Check sheet for the drawn part. Datum: minimum x, y, z corner. Units: mm. A direction names the side the tool comes from. Coordinates: 2 decimals unless noted, no trailing zeros. Order: outer loops, then holes, each group sorted by start corner. A loop starts at its lowest first (then second) coordinate and runs counter-clockwise, first axis right, second up. Notation, with made-up numbers: (9, -38.75) -> (57, -38.75) arc R13 cw to (57, -15.75) -> close; hole circle Ø11 at (32.5, -25). An arc over 180 degrees is marked (long way). Answer as CSV lines item,"result".
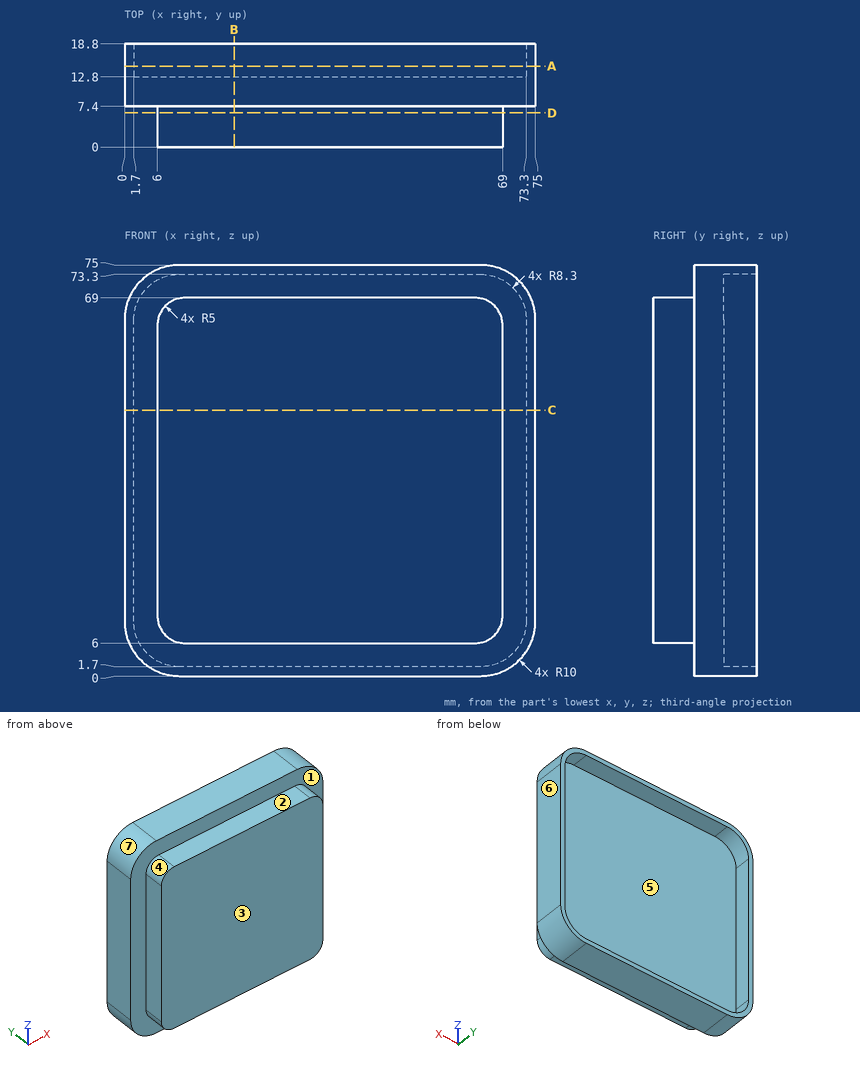
Item 1: Section check D-D, the plane y = 6.25. Record the boundary of the cut face in (x, z).
Answer list:
outline,"(6, 11) arc R5 ccw to (11, 6) -> (64, 6) arc R5 ccw to (69, 11) -> (69, 64) arc R5 ccw to (64, 69) -> (11, 69) arc R5 ccw to (6, 64) -> close"
Item 2: Section check A-A, the plane y = 14.75. Record the boundary of the cut face in (x, z), plus the area to 3 significant figures.
Answer list:
outline,"(0, 10) arc R10 ccw to (10, 0) -> (65, 0) arc R10 ccw to (75, 10) -> (75, 65) arc R10 ccw to (65, 75) -> (10, 75) arc R10 ccw to (0, 65) -> close; hole (1.7, 10) arc R8.3 ccw to (10, 1.7) -> (65, 1.7) arc R8.3 ccw to (73.3, 10) -> (73.3, 65) arc R8.3 ccw to (65, 73.3) -> (10, 73.3) arc R8.3 ccw to (1.7, 65) -> close"
area,"472 mm2"
Item 3: Depth check by flat-ended pin: pin 1 Ø8 at (y, z) = (3, 33.5) entering from -X; pin 2 Ø10 at (y, z) = (16, 21) entering from -X; pin 3 Ø1.5 at (x, z) = (50.5, 30.5) entering from +Y; pin 4 Ø3.5 at (x, y) = (39.5, 2.5) entering from +Z. Enter the tip coordinate at first touch or a pass-through.
Answer list:
pin 1,"x = 6"
pin 2,"x = 0"
pin 3,"y = 12.8"
pin 4,"z = 69"
Item 4: Section check B-B, the plane x = 20. Record the boundary of the cut face in (y, z).
Answer list:
outline,"(0, 6) -> (7.4, 6) -> (7.4, 0) -> (18.8, 0) -> (18.8, 1.7) -> (12.8, 1.7) -> (12.8, 73.3) -> (18.8, 73.3) -> (18.8, 75) -> (7.4, 75) -> (7.4, 69) -> (0, 69) -> close"
Item 5: Release check for a two-part mould opening along X. For the marked faces 5, 6 and 7 record: +X half, -X half, draft (parallel to the pull), parting line (faces both ways), or undercut.
Answer list:
face 5,"undercut"
face 6,"+X half"
face 7,"-X half"
Item 6: Tool access check on the marked faces 1, 2, 3 and 4. Record the directions out of +Z, -Z, +X, -X, +Y, -Y that give a thin tool (end or side, any length) a straight path to the whole face; none if there is none.
Answer list:
face 1,"-Y"
face 2,"+Z, +X, -X, -Y"
face 3,"+Z, -Z, +X, -X, -Y"
face 4,"+Z, -X, -Y"
Item 7: Section check C-C, the plane z = 48.5. Record the boundary of the cut face in (x, y), plus the area to 3 significant figures.
Answer list:
outline,"(0, 7.4) -> (6, 7.4) -> (6, 0) -> (69, 0) -> (69, 7.4) -> (75, 7.4) -> (75, 18.8) -> (73.3, 18.8) -> (73.3, 12.8) -> (1.7, 12.8) -> (1.7, 18.8) -> (0, 18.8) -> close"
area,"892 mm2"
Item 8: Thickness scan on line 1 (X direction, y = 15.5, z = 47); line 2 (Z direction, x = 41, y = 4). Record the ranges inside material, lowest first.
Answer list:
line 1,"0 to 1.7, 73.3 to 75"
line 2,"6 to 69"
